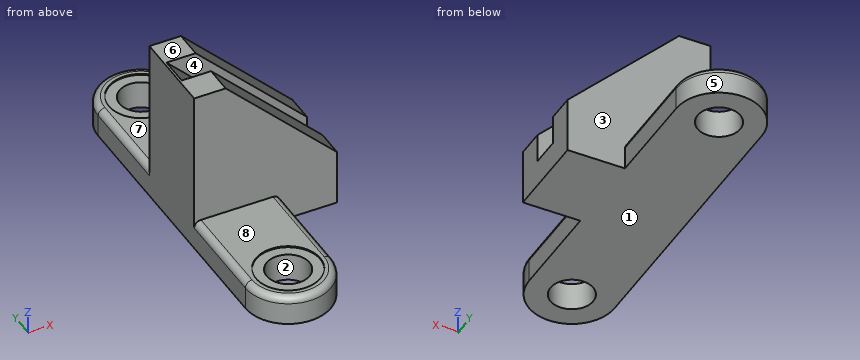
from build123d import *

# Parameters (mm, degrees)
F1_DEPTH  = 38
F4_DEPTH  = 13
F5_DEPTH  = 26
F6_R      = 19
F7_DEPTH  = 26.001
F8_R      = 28.5
F9_DEPTH  = 1
F10_R     = 19
F11_DEPTH = 26.001
F12_R     = 28.5
F13_DEPTH = 1
F14_R     = 6


with BuildPart() as f1:
    # F0 (on Front) → F1 (new body, symmetric)
    with BuildSketch(Plane.XZ):
        Polygon((0, 149), (0, 0), (127, 0), (127, 50), (28, 149), align=None)
    extrude(amount=F1_DEPTH, both=True)

    # F3 (on Front) → F4 (cut, symmetric)
    with BuildSketch(Plane.XZ):
        Polygon((127, 50), (28, 149), (2, 149), (127, 24), align=None)
    extrude(amount=F4_DEPTH, both=True, mode=Mode.SUBTRACT)

    # F2 (on face) → F5 (join)
    with BuildSketch(Plane(origin=(0, 0, 0), x_dir=(1, 0, 0), z_dir=(0, 0, -1))):
        with BuildLine():
            ThreePointArc((0, -125), (38, -163), (76, -125))
            Line((76, -125), (76, 125))
            ThreePointArc((76, 125), (38, 163), (0, 125))
            Line((0, 125), (0, -125))
        make_face()
    extrude(amount=-F5_DEPTH)

    # F6 (on face) → F7 (cut, through all)
    with BuildSketch(Plane.XY.offset(26)):
        with Locations((38, -125)):
            Circle(F6_R)
    extrude(amount=-F7_DEPTH, mode=Mode.SUBTRACT)

    # F8 (on face) → F9 (cut)
    with BuildSketch(Plane.XY.offset(26)):
        with Locations((38, -125)):
            Circle(F8_R)
    extrude(amount=-F9_DEPTH, mode=Mode.SUBTRACT)

    # F10 (on face) → F11 (cut, through all)
    with BuildSketch(Plane.XY.offset(26)):
        with Locations((38, 125)):
            Circle(F10_R)
    extrude(amount=-F11_DEPTH, mode=Mode.SUBTRACT)

    # F12 (on face) → F13 (cut)
    with BuildSketch(Plane.XY.offset(26)):
        with Locations((38, 125)):
            Circle(F12_R)
    extrude(amount=-F13_DEPTH, mode=Mode.SUBTRACT)

    # F14
    f14_edges = [f1.edges().sort_by_distance(p)[0] for p in [
        (76, -81.5, 26),
        (76, 81.5, 26),
        (0, 81.5, 26),
        (0, -81.5, 26),
        (38, -163, 26),
        (38, 163, 26),
    ]]
    fillet(f14_edges, radius=F14_R)


solid = f1.part
Work out the finished part from the listing and answer in its coordinate system (mm). Face numbers are marked on the shaded views. A direction names the side the tool comes from. Round coordinates to 2 decimals unless told otherwise and drop trailing zeros. Write each loop counter-clockwise with the first axis right and the second up, starting at its lowest first coordinate (ties: lowest second). Pieces come first, ordered by that corner, then holes.
1) A cutting plane is placed at B-B (z = 69). Give the vertices of the cut face in (x, y), plus the area to 3 significant figures.
2) The mould has two halves that part along Y. Classify the marked faces 1, 2 and 3: pulls with the +Y half, pulls with the -Y half, needs draft (parallel to the pull), parting line crosses it, or undercut.
3) Given pin 1 Ø1 at (x, z) = (26.5, 47) entering from +Y; pin 2 Ø10 at (x, y) = (81.5, -26) entering from +Z; pin 3 Ø6 at (x, z) = (99, 30) entering from -Y, each flat-ended and moving along its own axis, determine where each tip first touches the part or whether it passes through.
4) A tool of negligible diameter and unlimited length cuts with its end or side. For the marked faces 4, 5, 6, 7 and 8, from which of +Z, -Z, +X, -X, +Y, -Y can it reach the whole face along a straight path? Write none if from no direction.
5) A cutting plane is placed at A-A (x = 38). Give the number of separate pieces and of enclosed holes in the cut face, plus the area to 3 significant figures.
6) A cutting plane is placed at D-D (x = 91.5). Give the vertices of the cut face in (y, z), plus the area to 3 significant figures.
7) Straight lines are drawn through the part: line 1 (Y direction, x = 38, z = 10); line 2 (Y direction, x = 120.5, z = 56); line 3 (X direction, y = -51.5, z = 20.5). For each, find the intervals that lie inside material, in ascending order.
8) A cutting plane is placed at C-C (y = -111). Give the vertices of the cut face in (x, z), plus the area to 3 significant figures.
Completed:
1. outline: (0, -38) - (108, -38) - (108, -13) - (82, -13) - (82, 13) - (108, 13) - (108, 38) - (0, 38) - close
1. area: 7,530 mm2
2. face 1: needs draft
2. face 2: undercut
2. face 3: pulls with the +Y half
3. pin 1: stops at y = 38
3. pin 2: stops at z = 100.5
3. pin 3: stops at y = -38
4. face 4: +Z, +X
4. face 5: +Z, -Z, +Y
4. face 6: +Z, +X, -X, +Y, -Y
4. face 7: +Z, +X, -X, +Y
4. face 8: +Z, +X, -X, -Y
5. separate pieces: 3
5. enclosed holes: 0
5. area: 14,400 mm2
6. outline: (-38, 0) - (38, 0) - (38, 85.5) - (13, 85.5) - (13, 59.5) - (-13, 59.5) - (-13, 85.5) - (-38, 85.5) - close
6. area: 5,820 mm2
7. line 1: y = -163 to -144, -106 to 106, 144 to 163
7. line 2: y = -38 to -13, 13 to 38
7. line 3: x = 0.02 to 75.98
8. outline: (0, 0) - (25.15, 0) - (25.15, 25) - (13.18, 25) - (13.18, 26) - (6, 26) arc R6 ccw to (0, 20) - close; (50.85, 0) - (76, 0) - (76, 20) arc R6 ccw to (70, 26) - (62.82, 26) - (62.82, 25) - (50.85, 25) - close
8. area: 1,270 mm2
